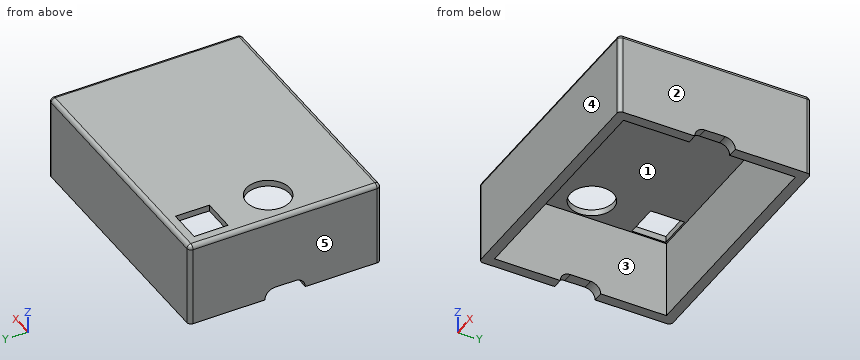
```python
from build123d import *

# Parameters (mm, degrees)
F0_W     = 127
F0_H     = 96.52
F0_R     = 10.922
F0_W_2   = 17.018
F0_H_2   = 17.018
F1_DEPTH = 3.175
F2_W     = 127
F2_H     = 96.52
F2_W_2   = 116.8399999365
F2_H_2   = 86.3599999365
F3_DEPTH = 39.37
F4_R     = 2.032
F5_W     = 5.0800000317
F5_H     = 20.32
F6_DEPTH = 5.08
F7_R     = 5.07999


# Not quite as in the source:
# - a fillet or chamfer is up to 0.001 mm smaller than in the source, because OpenCascade refuses the exact size


with BuildPart() as f1:
    # F0 (on Top) → F1 (new body)
    with BuildSketch(Plane.XY):
        with Locations((63.5, 48.26)):
            Rectangle(F0_W, F0_H)
        with Locations((16.764, 47.498)):
            Circle(F0_R, mode=Mode.SUBTRACT)
        with Locations((14.351, 82.169)):
            Rectangle(F0_W_2, F0_H_2, mode=Mode.SUBTRACT)
    extrude(amount=F1_DEPTH)

    # F2 (on face) → F3 (join)
    with BuildSketch(Plane(origin=(0, 0, 0), x_dir=(1, 0, 0), z_dir=(0, 0, -1))):
        with Locations((63.5, -48.26)):
            Rectangle(F2_W, F2_H)
        with Locations((63.5, -48.26)):
            Rectangle(F2_W_2, F2_H_2, mode=Mode.SUBTRACT)
    extrude(amount=F3_DEPTH)

    # F4
    f4_edges = [f1.edges().sort_by_distance(p)[0] for p in [
        (0, 96.52, -18.0975),
        (63.5, 96.52, 3.175),
        (0, 48.26, 3.175),
        (127, 96.52, -18.0975),
        (127, 48.26, 3.175),
        (127, 0, -18.0975),
        (63.5, 0, 3.175),
        (0, 0, -18.0975),
    ]]
    fillet(f4_edges, radius=F4_R)

    # F5 (on face) → F6 (cut)
    with BuildSketch(Plane(origin=(0, 0, -39.37), x_dir=(1, 0, 0), z_dir=(0, 0, -1))):
        with Locations((124.4599999841, -48.26)):
            Rectangle(F5_W, F5_H)
        with Locations((2.5400000159, -48.26)):
            Rectangle(F5_W, F5_H)
    extrude(amount=-F6_DEPTH, mode=Mode.SUBTRACT)

    # F7 (radius 5.08 in the source; OpenCascade refuses exactly that, so slightly less here)
    f7_edges = [f1.edges().sort_by_distance(p)[0] for p in [
        (2.54, 38.1, -34.29),
        (2.54, 58.42, -34.29),
        (124.46, 58.42, -34.29),
        (124.46, 38.1, -34.29),
    ]]
    fillet(f7_edges, radius=F7_R)


solid = f1.part
```
Verification items for the finished model (mm, model axes). Face numbers are marked on the shaded views. A direction names the side the tool comes from. Give positions to 0.01 mm unless a question says otherwise; leave off trailing zeros. Write each loop counter-clockwise with the first axis right and the second up, starting at its lowest first coordinate (ties: lowest second). Pieces come first, ordered by that corner, then holes. Notation, with made-up numbers: (37.25, -14) - (93.25, -14) arc R32 ccw to (93.25, 12) - close; hole circle Ø4 at (-30.5, -19). An arc over 180 degrees is marked (long way). Put each result on its own line as item: value.
Q1. Mould release check, pull along Y, two halves, no side actions. Record for the marked faces 3, 4 and 5: released by +Y, released by -Y, zero draft, split by the parting line, or undercut.
Result:
face 3: undercut
face 4: released by -Y
face 5: zero draft
Q2. Section check B-B on z = -15.5. Record the cut outline in (x, y).
Result:
outline: (0, 2.03) arc R2.03 ccw to (2.03, 0) - (124.97, 0) arc R2.03 ccw to (127, 2.03) - (127, 94.49) arc R2.03 ccw to (124.97, 96.52) - (2.03, 96.52) arc R2.03 ccw to (0, 94.49) - close; hole (5.08, 5.08) - (121.92, 5.08) - (121.92, 91.44) - (5.08, 91.44) - close
Q3. Depth check by flat-ended pin: P1, Ø4, axis at x = 106.5, y = 33, coming from the -Z side; P2, Ø1.5, axis at x = 2, y = 50, coming from the -Z side; P3, Ø17.5, axis at x = 16.764, y = 47.498, coming from the -Z side. Enter the tip coordinate at first touch or a pass-through.
Result:
P1: z = 0
P2: z = -34.29
P3: through
Q4. Section check A-A on y = 86. Record the cut outline in (x, z) (3 decimals).
Result:
outline: (0, -39.37) - (5.08, -39.37) - (5.08, 0) - (5.842, 0) - (5.842, 3.175) - (2.032, 3.175) arc R2.032 ccw to (0, 1.143) - close; (22.86, 0) - (121.92, 0) - (121.92, -39.37) - (127, -39.37) - (127, 1.143) arc R2.032 ccw to (124.968, 3.175) - (22.86, 3.175) - close
Q5. Scan lines: probe 1 along Y at (x, z) = (74, -8); probe 2 along X at (y, z) = (87, -13.5); probe 3 along X at (y, z) = (82, 0.5). Record each from-to range of solid material in increasing order. Write a range as from..to.
Result:
probe 1: 0..5.08, 91.44..96.52
probe 2: 0..5.08, 121.92..127
probe 3: 0..5.84, 22.86..127
Q6. Set-up check for the marked faces 1 and 2: record each of +Z, -Z, +X, -X, +Y, -Y from which the full face is reachable in a straight line by a thin tool's end or side.
Result:
face 1: -Z
face 2: +Z, -Z, +X, +Y, -Y
Q7. Section check C-C on x = 10. Record the cut outline in (y, z) (3 decimals).
Result:
outline: (0, -39.37) - (5.08, -39.37) - (5.08, 0) - (38.923, 0) - (38.923, 3.175) - (2.032, 3.175) arc R2.032 ccw to (0, 1.143) - close; (56.073, 0) - (73.66, 0) - (73.66, 3.175) - (56.073, 3.175) - close; (90.678, 0) - (91.44, 0) - (91.44, -39.37) - (96.52, -39.37) - (96.52, 1.143) arc R2.032 ccw to (94.488, 3.175) - (90.678, 3.175) - close
Q8. Section check D-D on x = 67.5. Record the cut outline in (y, z) (3 decimals), and give its area (3 significant figures).
Result:
outline: (0, -39.37) - (5.08, -39.37) - (5.08, 0) - (91.44, 0) - (91.44, -39.37) - (96.52, -39.37) - (96.52, 1.143) arc R2.032 ccw to (94.488, 3.175) - (2.032, 3.175) arc R2.032 ccw to (0, 1.143) - close
area: 705 mm2
